Source: CAD feature listing. Evaluate the final solid. Frame: model axes, mm. A direction names the side the tool comes from. Round coordinates to 2 decimals unless told otherwise and drop trailing zeros. Order: outer loops, then holes, each group sorted by start corner. A loop starts at its lowest first (then second) coordinate and runs counter-clockwise, first axis right, second up. Notation, with made-up numbers: (56, 85) - (97, 85) arc R22 cw to (97, 94) - close; hole circle Ø7 at (11, 56.5). An arc over 180 degrees is marked (long way). Put each result on its own line as item: value. Start each with the question number.
1) Section B-B on y = 5.75. Output: boundary loops of the cut face in (x, z).
2) Mould query, pull axis Z, two halves, no side actions, for faces 6 (the face through (-3.417, 16.233, -0.759)), 7 (the face through (-2, 7, -5)), 8 (the face through (-1, 15.1, -1)), 9 (the face through (13.66, 7.4, 2.74)). Classes: +Z half, -Z half, draft (parallel to the pull), parting line (faces both ways), or undercut.
3) Contact query for flat-ended pins moving along their axis: P1, Ø1.4, axis at x = 0.5, z = 0.5, coming from the -Y side; P2, Ø6, axis at x = 13, z = -2, coming from the +Y side; P3, Ø3, axis at x = 14.5, y = 7, coming from the +Z side. Output: stop coordinate, or through.
4) Section C-C on z = -5.25. Output: boundary loops of the cut face in (x, y), then the cut area to 3 significant figures.
5) Line query: probe 1 along X at (y, z) = (16.05, 0); probe 2 along Z at (x, y) = (19.5, 5.5); probe 3 along Y at (x, z) = (-1, 6). Output: solid intervals per line, ascending. Write a range as [from, to].
6) Section D-D on x = 16.5. Output: boundary loops of the cut face in (y, z), then the cut area to 3 significant figures.
7) Section A-A on z = 0. Output: boundary loops of the cut face in (x, y).
8) Access query for faces 1 (the face through (1, 1, 1)), 2 (the face through (2, 7, 5)), 3 (the face through (2, 7, -5)), 4 (the face through (0.736, 16.283, 2.337)), 5 (the face through (-2, 7, 5)). Directions: +Z, -Z, +X, -X, +Y, -Y. A direction counts if a zero-diameter tool reaches every point of the face in a straight line with its end or side. Return the directions, or none.
```python
from build123d import *

# Parameters (mm, degrees)
BOSS_EXTRUDE1_DEPTH = 15
SKETCH2_R           = 2.35
CUT_EXTRUDE1_DEPTH  = 1
SKETCH3_R           = 3.5
SKETCH3_R_2         = 2.45
BOSS_EXTRUDE2_DEPTH = 2.5
SKETCH4_R           = 1.2
CUT_EXTRUDE2_DEPTH  = 32.995663769
SKETCH5_R           = 2.45
SKETCH5_R_2         = 1.2
BOSS_EXTRUDE3_DEPTH = 0.1


with BuildPart() as part:
    # Sketch1 → Boss-Extrude1 (new body)
    with BuildSketch(Plane(origin=(0, 0, 0), x_dir=(1, 0, 0), z_dir=(0, 1, 0))):
        with BuildLine():
            Line((2, 6.35), (2, 3.5))
            Line((2, 3.5), (25, 2))
            ThreePointArc((25, 2), (27, 0), (25, -2))
            Line((25, -2), (2, -3.5))
            Line((2, -3.5), (2, -6.35))
            ThreePointArc((2, -6.35), (0, -8.35), (-2, -6.35))
            Line((-2, -6.35), (-2, -2.95))
            ThreePointArc((-2, -2.95), (-3.564056677, 0), (-2, 2.95))
            Line((-2, 2.95), (-2, 6.35))
            ThreePointArc((-2, 6.35), (0, 8.35), (2, 6.35))
        make_face()
    extrude(amount=BOSS_EXTRUDE1_DEPTH)

    # Sketch2 → Cut-Extrude1 (cut)
    with BuildSketch(Plane.XZ):
        with Locations(Location((0, 0, 0), (0, 0, 270))):
            Circle(SKETCH2_R)
    extrude(amount=-CUT_EXTRUDE1_DEPTH, mode=Mode.SUBTRACT)

    # Sketch3 → Boss-Extrude2 (add)
    with BuildSketch(Plane(origin=(0, 15, 0), x_dir=(1, 0, 0), z_dir=(0, 1, 0))):
        with Locations(Location((0, 0, 0), (0, 0, 270))):
            Circle(SKETCH3_R)
        with Locations(Location((0, 0, 0), (0, 0, 270))):
            Circle(SKETCH3_R_2, mode=Mode.SUBTRACT)
    extrude(amount=BOSS_EXTRUDE2_DEPTH)

    # Sketch4 → Cut-Extrude2 (cut, through all)
    with BuildSketch(Plane(origin=(0, 15, 0), x_dir=(1, 0, 0), z_dir=(0, 1, 0))):
        with Locations(Location((0, 0, 0), (0, 0, 270))):
            Circle(SKETCH4_R)
    extrude(amount=-CUT_EXTRUDE2_DEPTH, mode=Mode.SUBTRACT)

    # Sketch5 → Boss-Extrude3 (add)
    with BuildSketch(Plane(origin=(0, 15, 0), x_dir=(1, 0, 0), z_dir=(0, 1, 0))):
        with Locations(Location((0, 0, 0), (0, 0, 270))):
            Circle(SKETCH5_R)
        with Locations(Location((0, 0, 0), (0, 0, 270))):
            Circle(SKETCH5_R_2, mode=Mode.SUBTRACT)
    extrude(amount=BOSS_EXTRUDE3_DEPTH)


solid = part.part
```
Answer sheet:
1. outline: (-2, -6.35) arc R2 ccw to (2, -6.35) - (2, -3.5) - (25, -2) arc R2 ccw to (25, 2) - (2, 3.5) - (2, 6.35) arc R2 ccw to (-2, 6.35) - (-2, 2.95) arc R3.56 ccw to (-2, -2.95) - close; hole circle Ø2.4 at (0, 0)
2. face 6: parting line
2. face 7: draft
2. face 8: undercut
2. face 9: +Z half
3. P1: y = 1
3. P2: y = 15
3. P3: z = 2.78
4. outline: (-2, 0) - (2, 0) - (2, 15) - (-2, 15) - close
4. area: 60.0 mm^2
5. probe 1: [-3.5, -2.45], [2.45, 3.5]
5. probe 2: [-2.36, 2.36]
5. probe 3: [0, 15]
6. outline: (0, -2.55) - (15, -2.55) - (15, 2.55) - (0, 2.55) - close
6. area: 76.6 mm^2
7. outline: (-3.56, 0) - (-2.35, 0) - (-2.35, 1) - (-1.2, 1) - (-1.2, 15.1) - (-2.45, 15.1) - (-2.45, 17.5) - (-3.5, 17.5) - (-3.5, 15) - (-3.56, 15) - close; (1.2, 1) - (2.35, 1) - (2.35, 0) - (27, 0) - (27, 15) - (3.5, 15) - (3.5, 17.5) - (2.45, 17.5) - (2.45, 15.1) - (1.2, 15.1) - close
8. face 1: -Y
8. face 2: +Z, +X, +Y, -Y
8. face 3: -Z, +X, +Y, -Y
8. face 4: +Y
8. face 5: +Z, -X, +Y, -Y
